Geometry: final body of the model. Coordinates: model frame, mm. Face numbers are marked on the shaded views. A direction names the side the tool comes from. Round coordinates to 2 decimals unless told otherwise and drop trailing zeros. Loops run counter-clockwise (first coordinate to the right, second up) from the corner with the lowest first, then second, coordinate; pieces in that order, holes last. Notation, with made-up numbers: M 37.5,-3.5 L 74.5,-3.5 A16 cw 74.5,2.5 Z; hole C -38.5,80 d2. An arc over 180 degrees is marked long. Return JSON: item names as keys, results as strings.
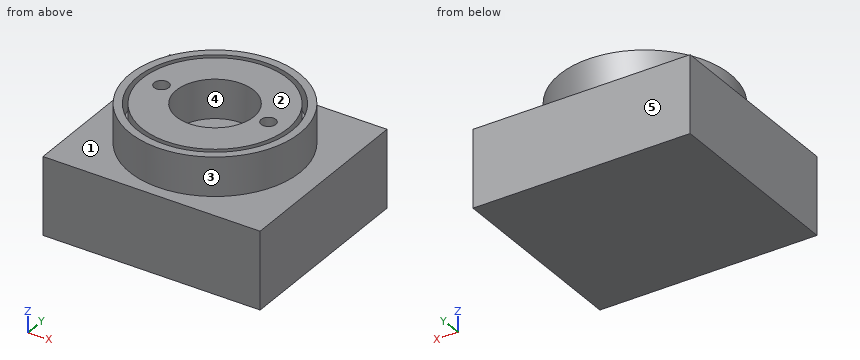
from build123d import *

# Parameters (mm, degrees)
BOSS_EXTRUDE1_DEPTH      = 10
BOSS_EXTRUDE1_DEPTH_BACK = 15
SKETCH1_R                = 55
SKETCH1_R_2              = 25
SKETCH2_R                = 50
SKETCH2_R_2              = 47
SKETCH2_R_3              = 4.75
CUT_EXTRUDE1_DEPTH       = 15
SKETCH4_W                = 140
SKETCH4_H                = 125
BOSS_EXTRUDE3_DEPTH      = 50


with BuildPart() as part:
    # Sketch1 → Boss-Extrude1 (new, two sides: drawn at the far end of the back side and taken through both)
    with BuildSketch(Plane.XY.offset(-BOSS_EXTRUDE1_DEPTH_BACK)):
        Circle(SKETCH1_R)
        Circle(SKETCH1_R_2, mode=Mode.SUBTRACT)
    extrude(amount=BOSS_EXTRUDE1_DEPTH + BOSS_EXTRUDE1_DEPTH_BACK)

    # Sketch2 → Cut-Extrude1 (cut)
    # profile 1 of 3: a face of its own
    with BuildSketch(Plane.XY.offset(10)):
        Circle(SKETCH2_R)
        Circle(SKETCH2_R_2, mode=Mode.SUBTRACT)
    # profile 2 of 3: a face of its own
    with BuildSketch(Plane.XY.offset(10)):
        with Locations((-34.5, 0)):
            Circle(SKETCH2_R_3)
    # profile 3 of 3: a face of its own
    with BuildSketch(Plane.XY.offset(10)):
        with Locations((34.5, 0)):
            Circle(SKETCH2_R_3)
    extrude(amount=-CUT_EXTRUDE1_DEPTH, mode=Mode.SUBTRACT)

    # Sketch4 → Boss-Extrude3 (add)
    with BuildSketch(Plane(origin=(0, 0, -15), x_dir=(-1, 0, 0), z_dir=(0, 0, -1))):
        Rectangle(SKETCH4_W, SKETCH4_H)
    extrude(amount=BOSS_EXTRUDE3_DEPTH)


solid = part.part
Q1. Section query C-C (z = -10.5). Output: boundary loops of the cut face in (x, y).
Determined:
{"outline": "C 0,0 d110; hole C 0,0 d50"}
Q2. Section query D-D (x = 34.5). Output: boundary loops of the cut face in (y, z), plus the area to 3 significant figures.
Determined:
{"outline": "M -62.5,-65 L 62.5,-65 L 62.5,-15 L 42.83,-15 L 42.83,10 L 36.19,10 L 36.19,-5 L 31.92,-5 L 31.92,10 L 4.75,10 L 4.75,-5 L -4.75,-5 L -4.75,10 L -31.92,10 L -31.92,-5 L -36.19,-5 L -36.19,10 L -42.83,10 L -42.83,-15 L -62.5,-15 Z", "area": "8,120 mm^2"}
Q3. Section query B-B (y = 0). Output: boundary loops of the cut face in (x, z), plus the area to 4 significant figures.
Determined:
{"outline": "M -70,-65 L 70,-65 L 70,-15 L 55,-15 L 55,10 L 50,10 L 50,-5 L 47,-5 L 47,10 L 39.25,10 L 39.25,-5 L 29.75,-5 L 29.75,10 L 25,10 L 25,-15 L -25,-15 L -25,10 L -29.75,10 L -29.75,-5 L -39.25,-5 L -39.25,10 L -47,10 L -47,-5 L -50,-5 L -50,10 L -55,10 L -55,-15 L -70,-15 Z", "area": "8,125 mm^2"}
Q4. Pull-direction query (X, two-part tool) for the marked faces 3, 4 and 5; classes: pulls with the +X half, pulls with the -X half, needs draft (parallel to the pull), parting line crosses it, or undercut.
Determined:
{"face 3": "parting line crosses it", "face 4": "undercut", "face 5": "needs draft"}
Q5. Section query A-A (x = 0). Output: boundary loops of the cut face in (y, z), plus the area to 3 significant figures.
Determined:
{"outline": "M -62.5,-65 L 62.5,-65 L 62.5,-15 L 55,-15 L 55,10 L 50,10 L 50,-5 L 47,-5 L 47,10 L 25,10 L 25,-15 L -25,-15 L -25,10 L -47,10 L -47,-5 L -50,-5 L -50,10 L -55,10 L -55,-15 L -62.5,-15 Z", "area": "7,660 mm^2"}
Q6. Material intervals for L1, parallel to Y at x = 0, z = 6; L2, parallel to Y at x = -34.5, z = -1.25; L3, parallel to X at y = -14, z = 2.5, sorted ascending.
Determined:
{"L1": "y = -55 to -50, -47 to -25, 25 to 47, 50 to 55", "L2": "y = -42.83 to -36.19, -31.92 to -4.75, 4.75 to 31.92, 36.19 to 42.83", "L3": "x = -53.19 to -48, -44.87 to -20.71, 20.71 to 44.87, 48 to 53.19"}
Q7. Pin query (flat end, axial travel): pin 1 (10 mm diameter, centred on x = 7, y = 1, fed in from +Z); pin 2 (3 mm diameter, centred on x = -36.5, y = 1.5, fed in from +Z); pin 3 (10 mm diameter, centred on x = 31, z = -3, fed in from -Y). Return the tip coordinate at first contact, or that it passes through.
Determined:
{"pin 1": "stops at z = -15", "pin 2": "stops at z = -5", "pin 3": "stops at y = -48.47"}
Q8. Reachability of the marked faces 1 and 2 from +Z, -Z, +X, -X, +Y, -Y: full face, straight path, thin tool, end or side. Return the list, or none.
Determined:
{"face 1": "+Z", "face 2": "+Z, +X, -X, +Y, -Y"}
